Build history of the part. All positions in model axes, mm. Round coordinates to 2 decimals unless told otherwise and drop trailing zeros. Write each loop counter-clockwise with the first axis right and the second up, starting at its lowest first coordinate (ties: lowest second). Pieces come first, ordered by that corner, then holes. Notation, with made-up numbers: M 83,76 L 130,76 A18 cw 130,90 Z; hole C 0,-17.5 d10. An arc over 180 degrees is marked long. Use a Markdown table: item, result.
from build123d import *

# Parameters (mm, degrees)
SKETCH_1_R      = 1.65
EXTRUDE_1_DEPTH = 3


with BuildPart() as part:
    # 草图1 → 凸台-拉伸1 (new body)
    with BuildSketch(Plane.XY):
        with BuildLine():
            ThreePointArc((-25, 0), (0, 25), (25, 0))
            ThreePointArc((25, 0), (35, -10), (45, 0))
            ThreePointArc((45, 0), (0, 45), (-45, 0))
            ThreePointArc((-45, 0), (-35, -10), (-25, 0))
        make_face()
        with Locations((-35, 0)):
            Circle(SKETCH_1_R, mode=Mode.SUBTRACT)
        with Locations((35, 0)):
            Circle(SKETCH_1_R, mode=Mode.SUBTRACT)
    extrude(amount=EXTRUDE_1_DEPTH)


solid = part.part
Q1. Drop flat-ended pins along their axis: P1, Ø1.5, axis at x = -5.5, z = 2, coming from the +Y side; P2, Ø1, axis at x = -29.5, z = 1.5, coming from the -Y side. Give the stop position or say it passes through.
Response values:
| item | result |
|---|---|
| P1 | stops at y = 44.75 |
| P2 | stops at y = -8.66 |
Q2. Two-plate mould, pull along X, no slides. Class faces 1 (the flat face through (-1, 30, 0)), 2 (the cylindrical face through (0.99, 44.99, 1.48)), 3 (the cylindrical face through (-35, -10, 1)): +X half, -X half, draft (parallel to the pull), parting line (faces both ways), or undercut.
Response values:
| item | result |
|---|---|
| face 1 | draft |
| face 2 | parting line |
| face 3 | undercut |
Q3. Cut at C-C on y = 16. Give the cut face in (x, z), and give its area (3 significant figures).
Response values:
| item | result |
|---|---|
| outline | M -42.06,0 L -19.21,0 L -19.21,3 L -42.06,3 Z; M 19.21,0 L 42.06,0 L 42.06,3 L 19.21,3 Z |
| area | 137 mm2 |
Q4. Cut at B-B on x = 35. Give the cut face in (y, z), and give its area (3 significant figures).
Response values:
| item | result |
|---|---|
| outline | M -10,0 L -1.65,0 L -1.65,3 L -10,3 Z; M 1.65,0 L 28.28,0 L 28.28,3 L 1.65,3 Z |
| area | 105 mm2 |
Q5. Drill centre lines: L1, parallel to X at y = -7, z = 2.45; L2, parallel to Y at x = 35, z = 1.75; L3, parallel to X at y = 17.5, z = 0.5. Where is each one in solid material? Low to high.
Response values:
| item | result |
|---|---|
| L1 | x = -42.14 to -27.86, 27.86 to 42.14 |
| L2 | y = -10 to -1.65, 1.65 to 28.28 |
| L3 | x = -41.46 to -17.85, 17.85 to 41.46 |
Q6. Cut at A-A on z = 1.65. Give the cut face in (x, y), and give its area (3 significant figures).
Response values:
| item | result |
|---|---|
| outline | M -45,0 A10 ccw -25,0 A25 cw 25,0 A10 ccw 45,0 A45 ccw Z; hole C -35,0 d3.3; hole C 35,0 d3.3 |
| area | 2,500 mm2 |
Q7. Cut at D-D on x = 0. Give the cut face in (y, z).
Response values:
| item | result |
|---|---|
| outline | M 25,0 L 45,0 L 45,3 L 25,3 Z |
